Could you check a few things on this drawing? It's one solid part, dimensions in mm from its lowest x, y, z. Coordinates: 2 decimals unless noted, no trailing zeros. Order: outer loops, then holes, each group sorted by start corner. A loop starts at its lowest first (then second) coordinate and runs counter-clockwise, first axis right, second up.
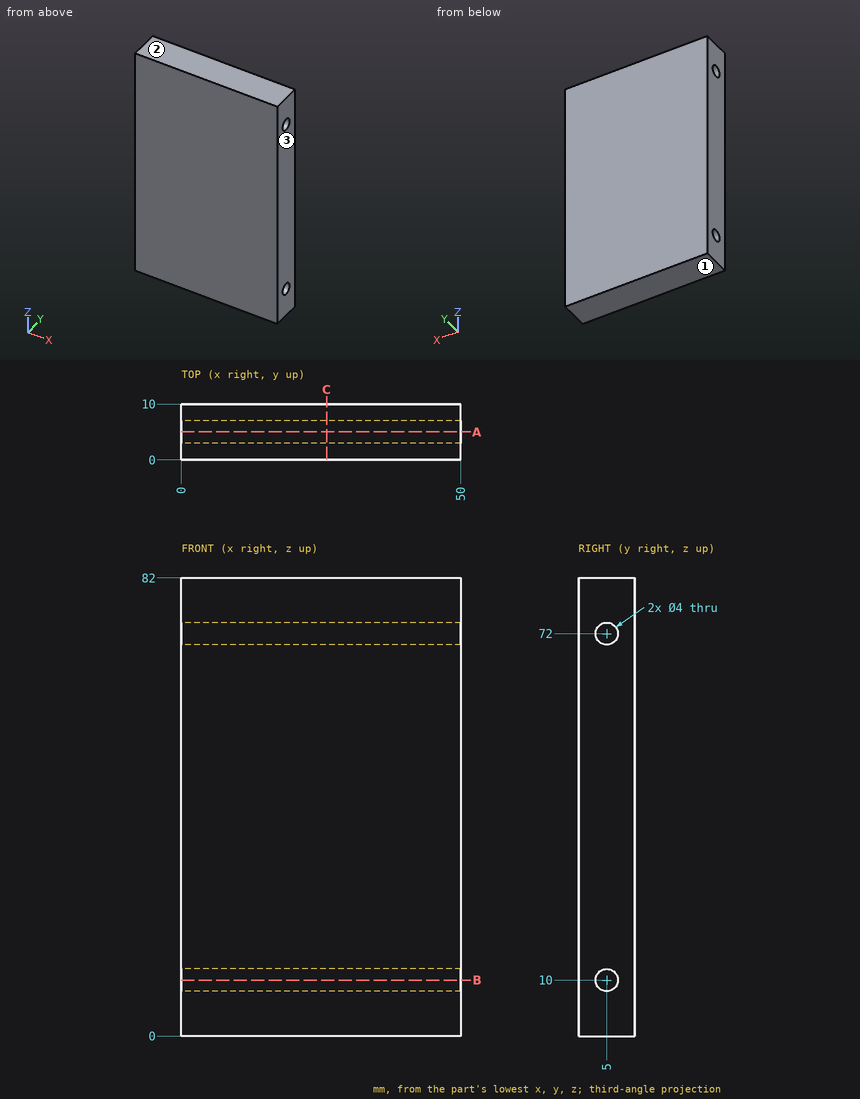
1. Imagine slicing it at B-B on z = 10. Please give me the cut outline in (x, y), then the cut area to 3 significant figures.
Completed:
outline: (0, 0) - (50, 0) - (50, 3) - (0, 3) - close; (0, 7) - (50, 7) - (50, 10) - (0, 10) - close
area: 300 mm2
2. I'm going to push a flat-ended pin straight in: pin 1 (3.5 mm diameter, centred on y = 5, z = 10, fed in from +X). Where does the tip first touch, or does it pass through?
Completed:
pin 1: passes through
3. Imagine slicing it at C-C on x = 26. Please give me the cut outline in (y, z), then the cut area to 3 significant figures.
Completed:
outline: (0, 0) - (10, 0) - (10, 82) - (0, 82) - close; hole circle Ø4 at (5, 10); hole circle Ø4 at (5, 72)
area: 795 mm2
4. Imagine slicing it at A-A on y = 5. Please give me the cut outline in (x, z).
Completed:
outline: (0, 0) - (50, 0) - (50, 8) - (0, 8) - close; (0, 12) - (50, 12) - (50, 70) - (0, 70) - close; (0, 74) - (50, 74) - (50, 82) - (0, 82) - close
5. Thinking about a two-plate mould opening in Z: for the marked faces 1, 2 and 3, which applies, pulls with the +Z half, pulls with the -Z half, needs draft (parallel to the pull), parting line crosses it, or undercut?
Completed:
face 1: pulls with the -Z half
face 2: pulls with the +Z half
face 3: needs draft
6. Please list where these lines run through material, in increasing order: probe 1 along Z at (x, y) = (37, 5); probe 2 along Y at (x, z) = (28, 10); probe 3 along Z at (x, y) = (23.5, 4.25).
Completed:
probe 1: z = 0 to 8, 12 to 70, 74 to 82
probe 2: y = 0 to 3, 7 to 10
probe 3: z = 0 to 8.15, 11.85 to 70.15, 73.85 to 82
